Autodesk Inventor part; units mm, degrees
ref_plane "Work Plane1" through (7, 0, 0) normal (-1, 0, 0) x (0, 0, 1)
ref_plane "YZ Plane" through (0, 0, 0) normal (1, 0, 0) x (0, 1, 0)
ref_plane "XZ Plane" through (0, 0, 0) normal (0, 1, 0) x (-1, 0, 0)
sketch "Sketch1" plane through (0, 0, 0) normal (1, 0, 0) x (0, 1, 0)
  arc A0 (26.1895, -3.5687) -> (0, 9.3537) centre (0, -23.6463) ccw
  arc A1 (17.8047, 26.4685) -> (0, 31.6837) centre (0, -1.3163) ccw
  line L0 (91.8773, 20.6837) -> (-78.3169, 20.6837)
  arc A2 (43.2558, 10.1592) -> (50, 33.1837) centre (50, 20.6837) ccw
  arc A3 (26.1895, -3.5687) -> (50, 44.6837) centre (49.9981, 14.6837) ccw
  line L1 (43.2558, 10.1592) -> (17.8047, 26.4685)
  line L2 (0, 54.8963) -> (0, -73.9166)
  line L3 (50, 20.6837) -> (50, 74.3533) construction
  line L4 (50, 44.6837) -> (50, 33.1837)
  arc A4 (34.7544, 43.9339) -> (34.7503, 33.9462) centre (35, 38.94) ccw
  line L5 (50, 44.6837) -> (34.7544, 43.9339)
  line L6 (50, 33.1837) -> (34.7503, 33.9462)
  point P0 (0, 0)
  point P1 (0, 20.6837)
  dimension "d0" = 66
  dimension "d1" = 66
  dimension "d2" = 22.33
  dimension "d3" = 22
  dimension "d4" = 25
  dimension "d5" = 50
  dimension "d6" = 60
  dimension "d7" = 6
  dimension "d8" = 10
  dimension "d9" = 15
extrude "Extrusion1" add sketch "Sketch1" along normal blind 14 contours A0 L2 L0 L1 A2 A3 | L0 A2 L4 A3 | L2 A1 L1 L0 | L4 L6 A4 L5
chamfer "Chamfer1" distance 2 angle 45 16 edges at (14, 76.901, 1.4083) (14, 14.602, 5.9473) (0, 76.901, 1.4083) (0, 14.602, 5.9473) (14, 42.3752, 33.565) (14, 30, 38.942) (14, 42.3772, 44.3088) (14, 61.996, 17.1699) (14, 30.5303, 18.3138) (14, 9.2764, 30.3531) (0, 42.3772, 44.3088) (0, 30, 38.942) (0, 42.3752, 33.565) (0, 30.5303, 18.3138) (0, 9.2764, 30.3531) (0, 61.996, 17.1699)
ref_plane "Work Plane1" through (7, 0, 0) normal (-1, 0, 0) x (0, 0, 1)
sketch "Sketch2" plane through (7, 0, 0) normal (-1, 0, 0) x (0, 0, 1)
  line L0 (29.6837, 0) -> (11.3537, 0)
  line L1 (26.5187, 0) -> (14.5187, 0)
  line L2 (26.5187, -29) -> (26.5187, -11.0524)
  line L3 (27.0187, -11.0524) -> (27.0187, -2)
  line L4 (29.0187, 0) -> (30.2528, 0)
  line L5 (12.0186, 0) -> (11.3537, 0)
  arc A0 (29.0187, 0) -> (27.0187, -2) centre (29.0187, -2) ccw
  line L6 (20.5187, -31.2918) -> (20.5187, 0)
  line L7 (29.0187, 0) -> (12.0186, 0)
  line L8 (27.0187, -11.0524) -> (26.5187, -11.0524)
  arc A1 (20.5187, -31.2918) -> (26.5187, -29) centre (20.7329, -22.8528) ccw
  line L9 (29.0187, 0) -> (20.5187, 0)
  point P0 (0, 0)
  point P1 (27.0187, 0)
  dimension "d19" = 0.5
  dimension "d20" = 2
  dimension "d21" = 6
  dimension "d22" = 31.2918
revolve "Revolution1" add sketch "Sketch2" angle 360 about axis through (7, -31.2918, 20.5187) along (0, 1, 0)
thread "Thread1"
thread "Thread2"
properties part number "Gancho"
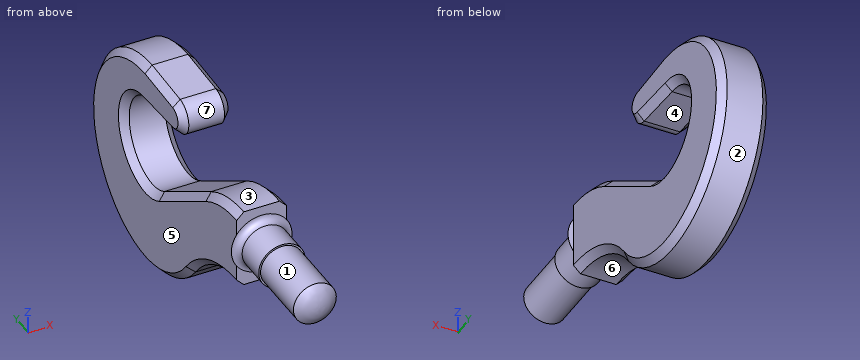
Here's how the part is built. I have some questions about the finished solid (model axes, mm). Face numbers are marked on the shaded views. A direction names the side the tool comes from. Round coordinates to 2 decimals unless told otherwise and drop trailing zeros. Order: outer loops, then holes, each group sorted by start corner. A loop starts at its lowest first (then second) coordinate and runs counter-clockwise, first axis right, second up. Notation, with made-up numbers: (80.25, 89) -> (123.25, 89) arc R26 cw to (123.25, 124) -> close; hole circle Ø2 at (62.25, 9). An arc over 180 degrees is marked (long way). Use a Markdown table: item, result. Add a question column.
(1) For pin 1 Ø1.5 at (x, y) = (3, 13) entering from +Z; pin 2 Ø4 at (x, z) = (9.5, 18) entering from -Y; pin 3 Ø8 at (x, y) = (10, 44) entering from +Z, each with a flat end and sliding along its axis, tell me the tip position at first contact or that it passes through.
(2) Suppose I cut it at A-A, the plane y = -22. Please give me the cut outline in (x, z), and give its area (3 significant figures).
(3) I need wall thicknesses on line 1 along Z through (x, y) = (1.5, 61); line 2 along Z through (x, y) = (5, 44.5); line 3 along Y through (x, z) = (13.75, 14). Which ranges of each line are inside material? Lowest first, please.
(4) If we mould it in two halves opening along Z, with no side actions, what happens to the marked faces 5, 6 and 7? For each: released by +Z, released by -Z, zero draft, split by the parting line, or undercut.
(5) For the marked faces 1, 2, 3 and 4, which set-ups out of +Z, -Z, +X, -X, +Y, -Y let a thin tool reach every point of the face, with its end or its side?
Verdict:
| question | item | result |
|---|---|---|
| 1 | pin 1 | z = 29.33 |
| 1 | pin 2 | y = -31.19 |
| 1 | pin 3 | z = 44.59 |
| 2 | outline | circle Ø12 at (7, 20.52) |
| 2 | area | 113 mm2 |
| 3 | line 1 | -12.69 to 13.76, 27.61 to 42.06 |
| 3 | line 2 | -14.81 to 9.46, 33.46 to 44.41 |
| 3 | line 3 | 0 to 34.02, 62.59 to 78.24 |
| 4 | face 5 | zero draft |
| 4 | face 6 | released by -Z |
| 4 | face 7 | undercut |
| 5 | face 1 | -Y |
| 5 | face 2 | +X, -X |
| 5 | face 3 | +Z, +X, -X |
| 5 | face 4 | +X, -X, -Y |
